from build123d import *

# Parameters (mm, degrees)
F0_R     = 12.7
F1_DEPTH = 88.9
F2_W     = 38.1
F2_H     = 12.7
F3_DEPTH = 101.6
F4_DEPTH = 50.8
F6_DEPTH = 50.801
F8_DEPTH = 88.901


with BuildPart() as f1:
    # F0 (on Right) → F1 (new body)
    with BuildSketch(Plane.YZ):
        Polygon((-101.6, 0), (0, 0), (0, 69.85), (-50.8, 69.85), (-101.6, 50.8), align=None)
        with Locations((-38.1, 31.75)):
            Circle(F0_R, mode=Mode.SUBTRACT)
    extrude(amount=F1_DEPTH)

    # F2 (on face) → F3 (cut)
    with BuildSketch(Plane(origin=(0, 0, 0), x_dir=(-1, 0, 0), z_dir=(0, 1, 0))):
        with Locations((-44.45, 63.5)):
            Rectangle(F2_W, F2_H)
    extrude(amount=-F3_DEPTH, mode=Mode.SUBTRACT)

    # F4 (add): a face of the model
    f4_faces = [f1.faces().sort_by_distance(p)[0] for p in [
        (44.45, -101.6, 25.4),
    ]]
    extrude(f4_faces, amount=F4_DEPTH)

    # F5 (on face) → F6 (cut, through all)
    with BuildSketch(Plane.XY.offset(50.8)):
        Polygon((0, -152.4), (50.8, -152.4), (0, -101.6), align=None)
    extrude(amount=-F6_DEPTH, mode=Mode.SUBTRACT)

    # F7 (on face) → F8 (cut, through all)
    with BuildSketch(Plane.YZ.offset(88.9)):
        Polygon((-152.4, 31.75), (-101.6, 50.8), (-152.4, 50.8), align=None)
    extrude(amount=-F8_DEPTH, mode=Mode.SUBTRACT)


solid = f1.part
Here's how the part is built. I have some questions about the finished solid (model axes, mm). A direction names the side the tool comes from. Coordinates: 2 decimals unless noted, no trailing zeros. Order: outer loops, then holes, each group sorted by start corner. A loop starts at its lowest first (then second) coordinate and runs counter-clockwise, first axis right, second up.
Item 1: If we section it at D-D on y = -62: List the corners of the cut face in (x, z) for me, plus the area to 3 significant figures.
Result sheet:
outline: (0, 0) - (88.9, 0) - (88.9, 65.65) - (63.5, 65.65) - (63.5, 57.15) - (25.4, 57.15) - (25.4, 65.65) - (0, 65.65) - close
area: 5,510 mm2
Item 2: If we section it at B-B on z = 24: List the corners of the cut face in (x, y) for me, plus the area to 3 significant figures.
Result sheet:
outline: (0, -101.6) - (50.8, -152.4) - (88.9, -152.4) - (88.9, -48.16) - (0, -48.16) - close; (0, -28.04) - (88.9, -28.04) - (88.9, 0) - (0, 0) - close
area: 10,500 mm2
Item 3: I need wall thicknesses on line 1 (Z direction, x = 25.5, y = -38.1); line 2 (Y direction, x = 62, z = 31); line 3 (X direction, y = -24, z = 62). Which ranges of each line are inside material? Lowest first, please.
Result sheet:
line 1: z = 0 to 19.05, 44.45 to 57.15
line 2: y = -152.4 to -50.78, -25.42 to 0
line 3: x = 0 to 25.4, 63.5 to 88.9
Item 4: If we mould it in two halves opening along Y, with no side actions, what happens to faces 1 (the face through (88.9, -58, 28)), 2 (the face through (44, 0, 34)), 3 (the face through (25.8, -127.4, 20.1)), 4 (the face through (43.828, -48.178, 24.022))? For each: +Y half, -Y half, draft (parallel to the pull), parting line (faces both ways), or undercut.
Result sheet:
face 1: draft
face 2: +Y half
face 3: -Y half
face 4: undercut
Item 5: For faces 5 (the face through (45, -42, 57.15)), 6 (the face through (76, -25, 69.85)), which set-ups out of +Z, -Z, +X, -X, +Y, -Y let a thin tool reach every point of the face, with its end or its side?
Result sheet:
face 5: +Z, +Y, -Y
face 6: +Z, +X, -X, +Y, -Y
Item 6: If we section it at A-A on y = -38.1: List the corners of the cut face in (x, z) for me, plus the area to 3 significant figures.
Result sheet:
outline: (0, 0) - (88.9, 0) - (88.9, 19.05) - (0, 19.05) - close; (0, 44.45) - (88.9, 44.45) - (88.9, 69.85) - (63.5, 69.85) - (63.5, 57.15) - (25.4, 57.15) - (25.4, 69.85) - (0, 69.85) - close
area: 3,470 mm2
Item 7: For P1, Ø1, axis at y = -23, z = 44.5, coming from the -X side; P2, Ø4, axis at x = 37.5, y = -103, coming from the +Z side (3 decimals); P3, Ø19, axis at x = 46.5, y = -51.5, coming from the +Z side; P4, Ø8, axis at y = -113, z = 32.5, coming from the -X side, each with a flat end and sliding along its axis, tell me the tip position at first contact or that it passes through.
Result sheet:
P1: stops at x = 0
P2: stops at z = 51.025
P3: stops at z = 57.15
P4: stops at x = 7.4
Item 8: If we section it at C-C on x = 36: List the corners of the cut face in (y, z) for me, plus the area to 3 significant figures.
Result sheet:
outline: (-137.6, 0) - (0, 0) - (0, 57.15) - (-84.67, 57.15) - (-137.6, 37.3) - close; hole circle Ø25.4 at (-38.1, 31.75)
area: 6,830 mm2
